For this review, take the finished solid that the model builds, in its own axes (mm). A direction names the side the tool comes from. Give positions to 0.01 mm unless a question says otherwise; leave off trailing zeros. Write each loop counter-clockwise with the first axis right and the second up, starting at its lowest first coordinate (ties: lowest second). Pieces come first, ordered by that corner, then holes. Notation, with made-up numbers: M -15,30.5 L 15,30.5 A37 cw 15,68.5 Z; hole C 8,41 d8. An arc over 180 degrees is marked long. Write item = value, one per line.
```python
from build123d import *

# Parameters (mm, degrees)
SKETCH1_W          = 7.874
SKETCH1_H          = 76.2
EXTRUDE1_DEPTH     = 88.9
SKETCH2_R          = 5.207
CUT_EXTRUDE1_DEPTH = 8.874
FILLET1_R          = 6.35
SKETCH3_W          = 7.874
SKETCH3_H          = 6.35
EXTRUDE2_DEPTH     = 7.874


with BuildPart() as part:
    # Sketch1 → Extrude1 (new body)
    with BuildSketch(Plane.XY):
        with Locations((3.937, 38.1)):
            Rectangle(SKETCH1_W, SKETCH1_H)
    extrude(amount=EXTRUDE1_DEPTH)

    # Sketch2 → Cut-Extrude1 (cut, through all)
    with BuildSketch(Plane.ZY):
        with Locations((60.325, 23.8125)):
            Circle(SKETCH2_R)
        with Locations((60.325, 42.8625)):
            Circle(SKETCH2_R)
        with Locations((60.325, 61.9125)):
            Circle(SKETCH2_R)
        with Locations((41.275, 33.3375)):
            Circle(SKETCH2_R)
        with Locations((41.275, 52.3875)):
            Circle(SKETCH2_R)
        with Locations((41.275, 14.2875)):
            Circle(SKETCH2_R)
    extrude(amount=-CUT_EXTRUDE1_DEPTH, mode=Mode.SUBTRACT)

    # Fillet1
    fillet1_edges = [part.edges().sort_by_distance(p)[0] for p in [
        (3.937, 76.2, 88.9),
        (3.937, 0, 88.9),
    ]]
    fillet(fillet1_edges, radius=FILLET1_R)

    # Sketch3 → Extrude2 (add)
    with BuildSketch(Plane.XY):
        with Locations((3.937, 15.875)):
            Rectangle(SKETCH3_W, SKETCH3_H)
    extrude(amount=-EXTRUDE2_DEPTH)


solid = part.part
```
1. We need section D-D, the plane y = 41. Write out the cut boundary in (x, z), then the cut area to 3 significant figures.
Responses:
outline = M 0,0 L 7.87,0 L 7.87,55.46 L 0,55.46 Z; M 0,65.19 L 7.87,65.19 L 7.87,88.9 L 0,88.9 Z
area = 623 mm2
2. The part is to be moulded in two halves that separate along Z. For faces 1 (the face through (4, 39, 88.9)), 2 (the face through (7.874, 38, 51)), 3 (the face through (3.88, 36.86, 37.44)), say which applies: +Z half, -Z half, draft (parallel to the pull), parting line (faces both ways), or undercut.
Responses:
face_1 = +Z half
face_2 = draft
face_3 = undercut
3. We need section C-C, the plane z = 64.5. Write out the cut boundary in (x, y), then the cut area to 3 significant figures.
Responses:
outline = M 0,0 L 7.87,0 L 7.87,20.7 L 0,20.7 Z; M 0,26.92 L 7.87,26.92 L 7.87,39.75 L 0,39.75 Z; M 0,45.97 L 7.87,45.97 L 7.87,58.8 L 0,58.8 Z; M 0,65.02 L 7.87,65.02 L 7.87,76.2 L 0,76.2 Z
area = 453 mm2
4. Insertion check: P1, Ø2.5, axis at x = 4, y = 42.5, coming from the -Z side. The pin has a flat end and moves straight along its axis. Give the tip position at first contact, or say it passes through.
Responses:
P1 = 0
5. We need section A-A, the plane y = 16. Write out the cut boundary in (x, z), then the cut area to 3 significant figures.
Responses:
outline = M 0,-7.87 L 7.87,-7.87 L 7.87,36.36 L 0,36.36 Z; M 0,46.19 L 7.87,46.19 L 7.87,88.9 L 0,88.9 Z
area = 685 mm2
6. Machinability: for faces 4 (the face through (3.88, 25.38, 65.29)), 5 (the face through (4, 19.05, -4)), 6 (the face through (4, 12.7, -4)), which of the approach directions +Z, -Z, +X, -X, +Y, -Y give a long, thin tool a straight path to every point of the face, cutting with its end or side? Answer none if there is none.
Responses:
face_4 = +X, -X
face_5 = -Z, +X, -X, +Y
face_6 = -Z, +X, -X, -Y
7. We need section B-B, the plane x = 5.5. Count the separate pieces of the cut face and the enclosed holes in it, then the cut area to 3 significant figures.
Responses:
separate_pieces = 1
enclosed_holes = 6
area = 6,300 mm2
8. For line 1 along Y through (x, z) = (4.5, 44); line 2 along Z through (x, y) = (1.75, 47); line 3 along Z through (x, y) = (7, 16), list the stretches that pass through material, from the lowest coordinate up. Write a range as from..to.
Responses:
line_1 = 0..9.85, 18.72..28.9, 37.77..47.95, 56.82..76.2
line_2 = 0..57.16, 63.49..88.9
line_3 = -7.87..36.36, 46.19..88.9
